Geometry check sheet. Reference: the model listing, model coordinates, mm. A direction names the side the tool comes from. Round coordinates to 2 decimals unless told otherwise and drop trailing zeros. Write each loop counter-clockwise with the first axis right and the second up, starting at its lowest first coordinate (ties: lowest second). Pieces come first, ordered by that corner, then holes. Notation, with made-up numbers: M 63.5,50 L 85.5,50 A14 cw 85.5,57 Z; hole C 31,-25 d9. An arc over 180 degrees is marked long. Put each result on its own line as item: value. Start each with the question number.
(1) Section check C-C on z = -66. Record the cut outline in (x, y), then the cut area to 3 significant figures.
(2) Tool access check on faces 4 (the flat face through (7, 0, -4)), 5 (the flat face through (4.18, 11, 0)), 6 (the flat face through (16, 9.639, 0)), 7 (the flat face through (17, 11, -5)), 8 (the flat face through (31.5, 6, -46)). Record the directions out of +Z, -Z, +X, -X, +Y, -Y that give a thin tool (end or side, any length) a straight path to the whole face; none if there is none.
(3) Section check B-B on x = -27. Record the cut outline in (y, z), then the cut area to 3 significant figures.
(4) Gauge pin test, flat ends, axial feed: pin 1 (8 mm diameter, centred on x = -11, z = 1, fed in from +Y); pin 2 (1.5 mm diameter, centred on x = -11, y = 1.5, fed in from -Z); pin 3 (6 mm diameter, centred on y = 4.5, z = -42.5, fed in from -X). Record the tip position at first contact, or that the pin passes through.
(5) Material ranges on probe 1 along X at (y, z) = (3, -13); probe 2 along Y at (x, z) = (5.5, -3); probe 3 along Z at (x, y) = (2.5, 2.25), recorded low to high.
(6) Section check A-A on x = 19.5. Record the cut outline in (y, z).
(7) Mould release check, pull along Y, two halves, no side actions. Record for faces 1 (the flat face through (-31.5, 1, 0)), 2 (the flat face through (-2, 3, 0)), 3 (the flat face through (29, 11.5, -28)): pulls with the +Y half, pulls with the -Y half, needs draft (parallel to the pull), parting line crosses it, or undercut.
from build123d import *

# Parameters (mm, degrees)
SKETCH_1_W          = 63
SKETCH_1_H          = 10
EXTRUDE_1_DEPTH     = 2
SKETCH_4_W          = 2
SKETCH_4_H          = 10
EXTRUDE_2_DEPTH     = 93
SKETCH_5_W          = 61
SKETCH_5_H          = 10
EXTRUDE_3_DEPTH     = 1
SKETCH_6_W          = 10
SKETCH_6_H          = 92
EXTRUDE_4_DEPTH     = 1
SKETCH_7_W          = 3
SKETCH_7_H          = 10
EXTRUDE_5_DEPTH     = 93
SKETCH_10_W         = 26.594312394
SKETCH_10_H         = 101.559656513
CUT_EXTRUDE_1_DEPTH = 93
SKETCH_11_W         = 3
SKETCH_11_H         = 103
EXTRUDE_6_DEPTH     = 1.5
SKETCH_12_W         = 10
SKETCH_12_H         = 3.861283188
EXTRUDE_7_DEPTH     = 20.32
SKETCH_13_W         = 10
SKETCH_13_H         = 3.861283188
EXTRUDE_8_DEPTH     = 4
SKETCH_14_W         = 24.32
SKETCH_14_H         = 10
CUT_EXTRUDE_2_DEPTH = 2


with BuildPart() as part:
    # 草图1 → 凸台-拉伸1 (new body)
    with BuildSketch(Plane(origin=(0, 0, 0), x_dir=(1, 0, 0), z_dir=(0, 1, 0))):
        Rectangle(SKETCH_1_W, SKETCH_1_H)
    extrude(amount=EXTRUDE_1_DEPTH)

    # 草图4 → 凸台-拉伸2 (add)
    with BuildSketch(Plane(origin=(0, 2, 0), x_dir=(1, 0, 0), z_dir=(0, 1, 0))):
        with Locations((30.5, 0)):
            Rectangle(SKETCH_4_W, SKETCH_4_H)
    extrude(amount=EXTRUDE_2_DEPTH)

    # 草图5 → 凸台-拉伸3 (add)
    with BuildSketch(Plane(origin=(0, 2, 0), x_dir=(1, 0, 0), z_dir=(0, 1, 0))):
        with Locations((-1, 0)):
            Rectangle(SKETCH_5_W, SKETCH_5_H)
    extrude(amount=EXTRUDE_3_DEPTH)

    # 草图6 → 凸台-拉伸4 (add)
    with BuildSketch(Plane.ZY.offset(-29.5)):
        with Locations((0, 49)):
            Rectangle(SKETCH_6_W, SKETCH_6_H)
    extrude(amount=EXTRUDE_4_DEPTH)

    # 草图7 → 凸台-拉伸5 (add)
    with BuildSketch(Plane(origin=(0, 0, -5), x_dir=(-1, 0, 0), z_dir=(0, 0, -1))):
        with Locations((-30, 5)):
            Rectangle(SKETCH_7_W, SKETCH_7_H)
    extrude(amount=EXTRUDE_5_DEPTH)

    # 草图10 → 切除-拉伸1 (cut)
    with BuildSketch(Plane.ZY.offset(-28.5)):
        with Locations((8.297156197, 60.779828257)):
            Rectangle(SKETCH_10_W, SKETCH_10_H)
    extrude(amount=-CUT_EXTRUDE_1_DEPTH, mode=Mode.SUBTRACT)

    # 草图11 → 凸台-拉伸6 (add)
    with BuildSketch(Plane(origin=(0, 10, 0), x_dir=(1, 0, 0), z_dir=(0, 1, 0))):
        with Locations((30, 46.5)):
            Rectangle(SKETCH_11_W, SKETCH_11_H)
    extrude(amount=EXTRUDE_6_DEPTH)

    # 草图12 → 凸台-拉伸7 (add)
    with BuildSketch(Plane.ZY.offset(-28.5)):
        with Locations((0, 9.569358406)):
            Rectangle(SKETCH_12_W, SKETCH_12_H)
    extrude(amount=EXTRUDE_7_DEPTH)

    # 草图13 → 凸台-拉伸8 (add)
    with BuildSketch(Plane.ZY.offset(-8.18)):
        with Locations((0, 9.569358406)):
            Rectangle(SKETCH_13_W, SKETCH_13_H)
    extrude(amount=EXTRUDE_8_DEPTH)

    # 草图14 → 切除-拉伸2 (cut)
    with BuildSketch(Plane.XZ.offset(-7.638716812)):
        with Locations((16.34, 0)):
            Rectangle(SKETCH_14_W, SKETCH_14_H)
    extrude(amount=-CUT_EXTRUDE_2_DEPTH, mode=Mode.SUBTRACT)


solid = part.part
Answers follow:
1. outline: M 28.5,0 L 31.5,0 L 31.5,11.5 L 28.5,11.5 Z
1. area: 34.5 mm^2
2. face 4: +Z, -Z, +X, -X, -Y
2. face 5: +Z, -Z, -X, +Y
2. face 6: +Z, -Z, -X
2. face 7: -Z, -X, +Y, -Y
2. face 8: +Z, -Z, +X, +Y, -Y
3. outline: M 0,-5 L 3,-5 L 3,5 L 0,5 Z
3. area: 30.0 mm^2
4. pin 1: stops at y = 3
4. pin 2: stops at z = -5
4. pin 3: stops at x = 28.5
5. probe 1: x = 28.5 to 31.5
5. probe 2: y = 0 to 3, 9.64 to 11.5
5. probe 3: z = -5 to 5
6. outline: M 0,-5 L 3,-5 L 3,5 L 0,5 Z; M 9.64,-5 L 11.5,-5 L 11.5,5 L 9.64,5 Z
7. face 1: needs draft
7. face 2: undercut
7. face 3: pulls with the +Y half
